Part model, mm, in its own coordinate system. A direction names the side the tool comes from. Coordinates: 2 decimals unless noted, no trailing zeros. Loops run counter-clockwise (first coordinate to the right, second up) from the corner with the lowest first, then second, coordinate; pieces in that order, holes last. Notation, with made-up numbers: M 25.25,76 L 36.25,76 A9 cw 36.25,80 Z; hole C 62,22 d11. An arc over 180 degrees is marked long. Use a Markdown table: item, result. Add a question column.
1) Band-saw the part on D-D (x = 16). List the corners of the cut face in (y, z), plus the area to 3 significant figures.
2) Pull direction X, two halves, no side cores. Call faces 1 (the cylindrical face through (3.186, 6.391, -0.028)), 2 (the flat face through (27, 40, 0)), 3 (the flat face through (55, 26, 0)), 4 (the flat face through (0, 20, 0)): released by +X, released by -X, zero draft, split by the parting line, or undercut.
3) Tool access for faces 5 (the flat face through (8, 0, 0)), 6 (the flat face through (7, 3, 2)), 7 (the flat face through (35, 12, 0)), 8 (the cylindrical face through (2.21, 7.56, -1.49)), 9 (the cylindrical face through (4.507, 1.246, 1.493)): list every direction of +Z, -Z, +X, -X, +Y, -Y with a clear straight run to the whole face (end or side of a thin tool).
4) Band-saw the part on A-A (y = 5). List the corners of the cut face in (x, z), plus the area to 3 significant figures.
5) Pin check, flat tips, straight feed: pin 1 Ø6 at (x, y) = (5, 5) entering from -Z; pin 2 Ø0.6 at (y, z) = (3.5, 0) entering from +X; pin 3 Ø1 at (x, y) = (27.5, 21.5) entering from +Z; pin 4 Ø1 at (x, z) = (41, -0.5) entering from -Y. Stop position of each tip, or through.
6) Band-saw the part on B-B (x = 5). List the corners of the cut face in (y, z).
7) Band-saw the part on C-C (y = 19). List the corners of the cut face in (x, z).
8) Wall check: probe 1 along Y at (x, z) = (5, 0.9); probe 2 along Z at (x, y) = (47, 28); probe 3 along Y at (x, z) = (15.5, -0.55). Give the ranges that are in metal, low to high. Write a range as from..to.
Autodesk Inventor part; units mm, degrees
ref_plane "YZ Plane" through (0, 0, 0) normal (1, 0, 0) x (0, 1, 0)
ref_plane "XZ Plane" through (0, 0, 0) normal (0, 1, 0) x (-1, 0, 0)
ref_plane "XY Plane" through (0, 0, 0) normal (0, 0, 1) x (1, 0, 0)
sketch "Sketch1" plane through (0, 0, 0) normal (0, 0, 1) x (1, 0, 0)
  line L0 (0, 40) -> (55, 40)
  line L1 (55, 40) -> (55, 12)
  line L2 (7.5, 0) -> (0, 0)
  line L3 (0, 0) -> (0, 40)
  circle A0 centre (5, 5) radius 2.286
  circle A1 centre (5, 5) radius 3.786
  line L4 (55, 12) -> (15, 12)
  line L5 (15, 12) -> (15, 0)
  line L6 (15, 0) -> (0, 0)
  point P0 (0, 0)
  dimension "d2" = 0
  dimension "d3" = 0
  dimension "d4" = 4.572
  dimension "d7" = 1.5
  dimension "d13" = 28
  dimension "d14" = 55
extrude "Extrusion1" add sketch "Sketch1" along normal mid plane 2 contours L0 L1 L4 L5 L6 L2 L3 | A1
extrude "Extrusion2" add sketch "Sketch1" along normal mid plane 4 contours A1
properties part number "gate"
Entries:
| question | item | result |
|---|---|---|
| 1 | outline | M 12,-1 L 40,-1 L 40,1 L 12,1 Z |
| 1 | area | 56.0 mm2 |
| 2 | face 1 | undercut |
| 2 | face 2 | zero draft |
| 2 | face 3 | released by +X |
| 2 | face 4 | released by -X |
| 3 | face 5 | +Z, -Z, +X, -X, -Y |
| 3 | face 6 | +Z, +X, -X, +Y, -Y |
| 3 | face 7 | +Z, -Z, +X, -Y |
| 3 | face 8 | -Z |
| 3 | face 9 | +Z |
| 4 | outline | M 0,-1 L 1.21,-1 L 1.21,-2 L 2.71,-2 L 2.71,2 L 1.21,2 L 1.21,1 L 0,1 Z; M 7.29,-2 L 8.79,-2 L 8.79,-1 L 15,-1 L 15,1 L 8.79,1 L 8.79,2 L 7.29,2 Z |
| 4 | area | 26.9 mm2 |
| 5 | pin 1 | z = -2 |
| 5 | pin 2 | x = 15 |
| 5 | pin 3 | z = 1 |
| 5 | pin 4 | y = 12 |
| 6 | outline | M 0,-1 L 1.21,-1 L 1.21,-2 L 2.71,-2 L 2.71,2 L 1.21,2 L 1.21,1 L 0,1 Z; M 7.29,-2 L 8.79,-2 L 8.79,-1 L 40,-1 L 40,1 L 8.79,1 L 8.79,2 L 7.29,2 Z |
| 7 | outline | M 0,-1 L 55,-1 L 55,1 L 0,1 Z |
| 8 | probe 1 | 0..2.71, 7.29..40 |
| 8 | probe 2 | -1..1 |
| 8 | probe 3 | 12..40 |
